The model under review builds one solid part; all positions refer to its coordinate system, in mm. Face numbers are marked on the shaded views. A direction names the side the tool comes from. Give positions to 0.01 mm unless a question says otherwise; leave off trailing zeros. Loops run counter-clockwise (first coordinate to the right, second up) from the corner with the lowest first, then second, coordinate; pieces in that order, holes last. Notation, with made-up numbers: (53, 3.25) -> (103, 3.25) arc R25 cw to (103, 29.25) -> close; hole circle Ø2 at (64, 66). An arc over 180 degrees is marked (long way). Write each question's results on one line, items separated by ' | '. Start each with the question number.
Q1. We need section D-D (z = 5.75). Write out the cut boundary in (x, y).
Q2. Wall thickness on L1, parallel to Y at x = -4, z = 3; L2, parallel to X at y = 9.25, z = 0: over which ranges is each line inside the solid? List them lowest first. Write a range as [from, to].
Q3. We need section C-C (y = 4.5). Write out the cut boundary in (x, z), plus the area to 3 significant figures.
Q4. We need section B-B (x = 0). Write out the cut boundary in (y, z).
Q5. Machinability: for the marked faces 1 and 2, which of the approach directions +Z, -Z, +X, -X, +Y, -Y give a long, thin tool a straight path to every point of the face, cutting with its end or side? Answer none if there is none.
Q6. Insertion check: pin 1 Ø6 at (x, y) = (4.5, 2.5) entering from +Z; pin 2 Ø1.5 at (y, z) = (3, 2.5) entering from +X; pin 3 Ø2 at (x, z) = (1, 1) entering from +Y; pin 4 Ø5 at (y, z) = (12.5, 2) entering from +X. Each pin has a flat end and moves straight along its axis. Give the tip position at first contact, or say it passes through.
Q7. We need section A-A (z = 0). Write out the cut boundary in (x, y).
Q8. Mouldability with a two-part tool opening along Y and no side actions: class the marked faces 3, 4 and 5 as released by +Y, released by -Y, zero draft, split by the parting line, or undercut.
from build123d import *

# Parameters (mm, degrees)
SKETCH_1_R          = 6.5
EXTRUDE_1_DEPTH     = 6.5
SKETCH_2_R          = 4.85
EXTRUDE_2_DEPTH     = 7
SKETCH_3_R          = 6.5
EXTRUDE_3_DEPTH     = 0.5
SKETCH_4_R          = 2.5
CUT_EXTRUDE_1_DEPTH = 15


with BuildPart() as part:
    # 草图1 → 凸台-拉伸1 (new body)
    with BuildSketch(Plane(origin=(0, 0, 0), x_dir=(1, 0, 0), z_dir=(0, 1, 0))):
        Circle(SKETCH_1_R)
    extrude(amount=EXTRUDE_1_DEPTH)

    # 草图2 → 凸台-拉伸2 (add)
    with BuildSketch(Plane(origin=(0, 6.5, 0), x_dir=(1, 0, 0), z_dir=(0, 1, 0))):
        Circle(SKETCH_2_R)
    extrude(amount=EXTRUDE_2_DEPTH)

    # 草图3 → 凸台-拉伸3 (add)
    with BuildSketch(Plane(origin=(0, 13.5, 0), x_dir=(1, 0, 0), z_dir=(0, 1, 0))):
        Circle(SKETCH_3_R)
    extrude(amount=EXTRUDE_3_DEPTH)

    # 草图4 → 切除-拉伸1 (cut, through all)
    with BuildSketch(Plane(origin=(0, 14, 0), x_dir=(1, 0, 0), z_dir=(0, 1, 0))):
        Circle(SKETCH_4_R)
    extrude(amount=-CUT_EXTRUDE_1_DEPTH, mode=Mode.SUBTRACT)


solid = part.part
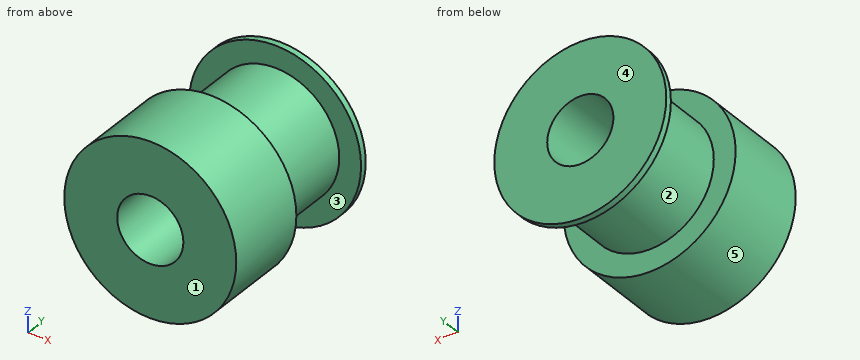
Output:
1) outline: (-3.03, 0) -> (3.03, 0) -> (3.03, 6.5) -> (-3.03, 6.5) -> close; (-3.03, 13.5) -> (3.03, 13.5) -> (3.03, 14) -> (-3.03, 14) -> close
2) L1: [0, 6.5], [13.5, 14] | L2: [-4.85, -2.5], [2.5, 4.85]
3) outline: circle Ø13 at (0, 0); hole circle Ø5 at (0, 0) | area: 113 mm2
4) outline: (0, -6.5) -> (6.5, -6.5) -> (6.5, -4.85) -> (13.5, -4.85) -> (13.5, -6.5) -> (14, -6.5) -> (14, -2.5) -> (0, -2.5) -> close; (0, 2.5) -> (14, 2.5) -> (14, 6.5) -> (13.5, 6.5) -> (13.5, 4.85) -> (6.5, 4.85) -> (6.5, 6.5) -> (0, 6.5) -> close
5) face 1: +Z, -Z, +X, -X, -Y | face 2: none
6) pin 1: z = 6.32 | pin 2: x = 6.26 | pin 3: through | pin 4: x = 6.5
7) outline: (-6.5, 0) -> (-2.5, 0) -> (-2.5, 14) -> (-6.5, 14) -> (-6.5, 13.5) -> (-4.85, 13.5) -> (-4.85, 6.5) -> (-6.5, 6.5) -> close; (2.5, 0) -> (6.5, 0) -> (6.5, 6.5) -> (4.85, 6.5) -> (4.85, 13.5) -> (6.5, 13.5) -> (6.5, 14) -> (2.5, 14) -> close
8) face 3: undercut | face 4: released by +Y | face 5: zero draft
